Input: part model. Units: mm. Frame: model coordinates. A direction names the side the tool comes from. Coordinates: 2 decimals unless noted, no trailing zeros. Order: outer loops, then holes, each group sorted by start corner. A loop starts at its lowest first (then second) coordinate and runs counter-clockwise, first axis right, second up. Notation, with made-up numbers: (-37.5, 11.5) -> (-19.5, 11.5) arc R15 cw to (-19.5, 23.5) -> close; hole circle Ø6 at (2, -19). An arc over 180 degrees is marked (long way). Use one line per item in the form item = value. Start each with the question number.
1) Pin query (flat end, axial travel): pin 1 (6 mm diameter, centred on y = -9, z = -21, fed in from -X); pin 2 (2 mm diameter, centred on y = -153, z = -19.5, fed in from +X); pin 3 (10 mm diameter, centred on x = -483, z = -46.5, fed in from -Y). Return the tip coordinate at first contact, or that it passes through.
2) Draft query along Z for faces 1 (the flat face through (14, -210, -75)), 2 (the flat face through (-922, -260, 34)), 3 (the flat face through (14, 240, -59)). Return one class per face: pulls with the +Z half, pulls with the -Z half, needs draft (parallel to the pull), parting line crosses it, or undercut.
3) Access query for faces 4 (the cylindrical face through (947.69, 209.58, 15.02)), 5 (the flat face through (14, 210, -65)), 6 (the flat face through (-1000, -246, 1)). Directions: +Z, -Z, +X, -X, +Y, -Y. A direction counts if a zero-diameter tool reaches every point of the face in a straight line with its end or side. Return the directions, or none.
4) Section query A-A on x = -756.5. Output: boundary loops of the cut face in (y, z), then the cut area to 3 significant figures.
5) Ray query, line 1 along Z through (x, y) = (0, 193); line 2 along Y through (x, z) = (368, 63); line 3 along X through (y, z) = (-62, 0). Return the intervals inside material, ascending.
6) Section query C-C on z = 0. Count the separate pieces of the cut face and the enclosed holes in it, then the cut area to 3 significant figures.
7) Section query B-B on y = -64. Output: boundary loops of the cut face in (x, z), then the cut area to 3 significant figures.
from build123d import *

# Parameters (mm, degrees)
F0_W          = 60
F0_H          = 130
F1_DEPTH      = 1000
F2_R          = 50
F2_R_2        = 40
F3_DEPTH      = 250
F3_DEPTH_BACK = 250
F4_DEPTH      = 250.001
F4_DEPTH_BACK = 250.001
F5_START      = 250
F5_DEPTH      = 10


with BuildPart() as f1:
    # F0 (on Right) → F1 (new body, symmetric)
    with BuildSketch(Plane.YZ):
        with BuildLine():
            Line((-240, -75), (-180, -75))
            ThreePointArc((-180, -75), (-172.9289321881, -72.0710678119), (-170, -65))
            Line((-170, -65), (-170, 65))
            ThreePointArc((-170, 65), (-172.9289321881, 72.0710678119), (-180, 75))
            Line((-180, 75), (-240, 75))
            ThreePointArc((-240, 75), (-247.0710678119, 72.0710678119), (-250, 65))
            Line((-250, 65), (-250, -65))
            ThreePointArc((-250, -65), (-247.0710678119, -72.0710678119), (-240, -75))
        make_face()
        with Locations((-210, 0)):
            Rectangle(F0_W, F0_H, mode=Mode.SUBTRACT)
    extrude(amount=F1_DEPTH, both=True)



with BuildPart() as f1b:
    # F0 (on Right) → F1, piece 2 (new body, symmetric)
    with BuildSketch(Plane.YZ):
        with BuildLine():
            ThreePointArc((250, 65), (247.0710678119, 72.0710678119), (240, 75))
            Line((240, 75), (180, 75))
            ThreePointArc((180, 75), (172.9289321881, 72.0710678119), (170, 65))
            Line((170, 65), (170, -65))
            ThreePointArc((170, -65), (172.9289321881, -72.0710678119), (180, -75))
            Line((180, -75), (240, -75))
            ThreePointArc((240, -75), (247.0710678119, -72.0710678119), (250, -65))
            Line((250, -65), (250, 65))
        make_face()
        with Locations((210, 0)):
            Rectangle(F0_W, F0_H, mode=Mode.SUBTRACT)
    extrude(amount=F1_DEPTH, both=True)


with BuildPart() as f1_1:
    add(f1.part)

    add(f1b.part)  # F3 merges F1b
    # F2 (on Front) → F3 (join, two sides)
    with BuildSketch(Plane.XZ) as f3_sk:
        with Locations((900, 0)):
            Circle(F2_R)
        with Locations((900, 0)):
            Circle(F2_R_2, mode=Mode.SUBTRACT)
        Circle(F2_R)
        Circle(F2_R_2, mode=Mode.SUBTRACT)
        with Locations((-900, 0)):
            Circle(F2_R)
        with Locations((-900, 0)):
            Circle(F2_R_2, mode=Mode.SUBTRACT)
    extrude(amount=F3_DEPTH)
    extrude(f3_sk.sketch, amount=-F3_DEPTH_BACK)

    # F2 (on Front) → F4 (cut, two sides)
    with BuildSketch(Plane.XZ) as f4_sk:
        with Locations((900, 0)):
            Circle(F2_R_2)
        Circle(F2_R_2)
        with Locations((-900, 0)):
            Circle(F2_R_2)
    extrude(amount=-F4_DEPTH, mode=Mode.SUBTRACT)
    extrude(f4_sk.sketch, amount=F4_DEPTH_BACK, mode=Mode.SUBTRACT)

    # F2 (on Front) → F5 (join)
    with BuildSketch(Plane.XZ.offset(F5_START)):
        with Locations((-900, 0)):
            Circle(F2_R)
        with Locations((-900, 0)):
            Circle(F2_R_2, mode=Mode.SUBTRACT)
    extrude(amount=F5_DEPTH)


solid = f1_1.part
Answers below:
q1.pin_1 = -946.65
q1.pin_2 = 946.45
q1.pin_3 = -250
q2.face_1 = pulls with the -Z half
q2.face_2 = needs draft
q2.face_3 = undercut
q3.face_4 = none
q3.face_5 = +X, -X
q3.face_6 = +Z, -Z, -X, +Y, -Y
q4.outline = (-250, -65) arc R10 ccw to (-240, -75) -> (-180, -75) arc R10 ccw to (-170, -65) -> (-170, 65) arc R10 ccw to (-180, 75) -> (-240, 75) arc R10 ccw to (-250, 65) -> close; (170, -65) arc R10 ccw to (180, -75) -> (240, -75) arc R10 ccw to (250, -65) -> (250, 65) arc R10 ccw to (240, 75) -> (180, 75) arc R10 ccw to (170, 65) -> close; hole (-240, -65) -> (-180, -65) -> (-180, 65) -> (-240, 65) -> close; hole (180, -65) -> (240, -65) -> (240, 65) -> (180, 65) -> close
q4.area = 8,230 mm^2
q5.line_1 = -75 to -65, -50 to -40, 40 to 50, 65 to 75
q5.line_2 = -250 to -240, -180 to -170, 170 to 180, 240 to 250
q5.line_3 = -950 to -940, -860 to -850, -50 to -40, 40 to 50, 850 to 860, 940 to 950
q6.separate_pieces = 4
q6.enclosed_holes = 6
q6.area = 98,200 mm^2
q7.outline = circle Ø100 at (-900, 0); circle Ø100 at (0, 0); circle Ø100 at (900, 0); hole circle Ø80 at (-900, 0); hole circle Ø80 at (0, 0); hole circle Ø80 at (900, 0)
q7.area = 8,480 mm^2
